```python
from build123d import *
from build123d.topology import SkipClean

# Parameters (mm, degrees)
SKETCH1_W           = 84
SKETCH1_H           = 40
BOSS_EXTRUDE1_DEPTH = 20
FILLET1_R           = 2
HOLE1_D             = 13
HOLE2_D             = 6
CUT_EXTRUDE2_DEPTH  = 17
RIB1_REACH          = 63.351
SKETCH10_WALLS_W    = 2
SKETCH10_WALLS_H    = 158.702893202
SKETCH12_W          = 3
SKETCH12_H          = 20
CUT_EXTRUDE3_DEPTH  = 60.439044407


with BuildPart() as part:
    # Sketch1 → Boss-Extrude1 (new, symmetric)
    with BuildSketch(Plane.XY):
        Rectangle(SKETCH1_W, SKETCH1_H)
    extrude(amount=BOSS_EXTRUDE1_DEPTH, both=True)

    # Fillet1
    fillet1_edges = [part.edges().sort_by_distance(p)[0] for p in [
        (42, -20, 0),
        (-42, -20, 0),
        (-42, 20, 0),
        (42, 20, 0),
    ]]
    fillet(fillet1_edges, radius=FILLET1_R)

    # Hole1 (through all)
    with Locations(Plane(origin=(0, 20, 0), x_dir=(1, 0, 0), z_dir=(0, 1, 0))):
        with Locations((0, 0)):
            Hole(HOLE1_D / 2)

    # Hole2 (through all)
    with Locations(Plane(origin=(0, 20, 0), x_dir=(1, 0, 0), z_dir=(0, 1, 0))):
        with Locations((12.5, 0), (0, -12.5), (-12.5, 0), (0, 12.5), (0, 0)):
            Hole(HOLE2_D / 2)

    # Sketch9 → Cut-Extrude2 (cut, symmetric)
    with BuildSketch(Plane(origin=(0, 0, 0), x_dir=(1, 0, 0), z_dir=(0, 1, 0))):
        with BuildLine():
            Line((-39, -20), (0, -20))
            Line((0, -20), (0, -18.5))
            ThreePointArc((0, -18.5), (-2.296100594, -18.043277195), (-4.242640687, -16.742640687))
            Line((-4.242640687, -16.742640687), (-16.742640687, -4.242640687))
            ThreePointArc((-16.742640687, -4.242640687), (-18.043277195, -2.296100594), (-18.5, 0))
            Line((-18.5, 0), (-39, 0))
            Line((-39, 0), (-39, -20))
        make_face()
        with BuildLine():
            Line((39, 0), (18.5, 0))
            ThreePointArc((18.5, 0), (18.043277195, -2.296100594), (16.742640687, -4.242640687))
            Line((16.742640687, -4.242640687), (4.242640687, -16.742640687))
            ThreePointArc((4.242640687, -16.742640687), (2.296100594, -18.043277195), (0, -18.5))
            Line((0, -18.5), (0, -20))
            Line((0, -20), (39, -20))
            Line((39, -20), (39, 0))
        make_face()
    extrude(amount=CUT_EXTRUDE2_DEPTH, both=True, mode=Mode.SUBTRACT)

    # Sketch10 walls → Rib1 (add, up to next)
    with BuildSketch(Plane.XY.offset(20), mode=Mode.PRIVATE) as rib1_sk1:
        Rectangle(SKETCH10_WALLS_W, SKETCH10_WALLS_H)
    rib1_tool1 = extrude(rib1_sk1.sketch, amount=-RIB1_REACH, mode=Mode.PRIVATE) - part.part
    # Sketch10 walls → Rib1 (add, up to next)
    with BuildSketch(Plane.XY.offset(20), mode=Mode.PRIVATE) as rib1_sk2:
        with Locations((5, 0)):
            Rectangle(SKETCH10_WALLS_W, SKETCH10_WALLS_H)
    rib1_tool2 = extrude(rib1_sk2.sketch, amount=-RIB1_REACH, mode=Mode.PRIVATE) - part.part
    # Sketch10 walls → Rib1 (add, up to next)
    with BuildSketch(Plane.XY.offset(20), mode=Mode.PRIVATE) as rib1_sk3:
        with Locations((10, 0)):
            Rectangle(SKETCH10_WALLS_W, SKETCH10_WALLS_H)
    rib1_tool3 = extrude(rib1_sk3.sketch, amount=-RIB1_REACH, mode=Mode.PRIVATE) - part.part
    # Sketch10 walls → Rib1 (add, up to next)
    with BuildSketch(Plane.XY.offset(20), mode=Mode.PRIVATE) as rib1_sk4:
        with Locations((15, 0)):
            Rectangle(SKETCH10_WALLS_W, SKETCH10_WALLS_H)
    rib1_tool4 = extrude(rib1_sk4.sketch, amount=-RIB1_REACH, mode=Mode.PRIVATE) - part.part
    # Sketch10 walls → Rib1 (add, up to next)
    with BuildSketch(Plane.XY.offset(20), mode=Mode.PRIVATE) as rib1_sk5:
        with Locations((20, 0)):
            Rectangle(SKETCH10_WALLS_W, SKETCH10_WALLS_H)
    rib1_tool5 = extrude(rib1_sk5.sketch, amount=-RIB1_REACH, mode=Mode.PRIVATE) - part.part
    # Sketch10 walls → Rib1 (add, up to next)
    with BuildSketch(Plane.XY.offset(20), mode=Mode.PRIVATE) as rib1_sk6:
        with Locations((25, 0)):
            Rectangle(SKETCH10_WALLS_W, SKETCH10_WALLS_H)
    rib1_tool6 = extrude(rib1_sk6.sketch, amount=-RIB1_REACH, mode=Mode.PRIVATE) - part.part
    # Sketch10 walls → Rib1 (add, up to next)
    with BuildSketch(Plane.XY.offset(20), mode=Mode.PRIVATE) as rib1_sk7:
        with Locations((30, 0)):
            Rectangle(SKETCH10_WALLS_W, SKETCH10_WALLS_H)
    rib1_tool7 = extrude(rib1_sk7.sketch, amount=-RIB1_REACH, mode=Mode.PRIVATE) - part.part
    # Sketch10 walls → Rib1 (add, up to next)
    with BuildSketch(Plane.XY.offset(20), mode=Mode.PRIVATE) as rib1_sk8:
        with Locations((35, 0)):
            Rectangle(SKETCH10_WALLS_W, SKETCH10_WALLS_H)
    rib1_tool8 = extrude(rib1_sk8.sketch, amount=-RIB1_REACH, mode=Mode.PRIVATE) - part.part
    # Sketch10 walls → Rib1 (add, up to next)
    with BuildSketch(Plane.XY.offset(20), mode=Mode.PRIVATE) as rib1_sk9:
        with Locations((-25, 0)):
            Rectangle(SKETCH10_WALLS_W, SKETCH10_WALLS_H)
    rib1_tool9 = extrude(rib1_sk9.sketch, amount=-RIB1_REACH, mode=Mode.PRIVATE) - part.part
    # Sketch10 walls → Rib1 (add, up to next)
    with BuildSketch(Plane.XY.offset(20), mode=Mode.PRIVATE) as rib1_sk10:
        with Locations((-20, 0)):
            Rectangle(SKETCH10_WALLS_W, SKETCH10_WALLS_H)
    rib1_tool10 = extrude(rib1_sk10.sketch, amount=-RIB1_REACH, mode=Mode.PRIVATE) - part.part
    # Sketch10 walls → Rib1 (add, up to next)
    with BuildSketch(Plane.XY.offset(20), mode=Mode.PRIVATE) as rib1_sk11:
        with Locations((-15, 0)):
            Rectangle(SKETCH10_WALLS_W, SKETCH10_WALLS_H)
    rib1_tool11 = extrude(rib1_sk11.sketch, amount=-RIB1_REACH, mode=Mode.PRIVATE) - part.part
    # Sketch10 walls → Rib1 (add, up to next)
    with BuildSketch(Plane.XY.offset(20), mode=Mode.PRIVATE) as rib1_sk12:
        with Locations((-10, 0)):
            Rectangle(SKETCH10_WALLS_W, SKETCH10_WALLS_H)
    rib1_tool12 = extrude(rib1_sk12.sketch, amount=-RIB1_REACH, mode=Mode.PRIVATE) - part.part
    # Sketch10 walls → Rib1 (add, up to next)
    with BuildSketch(Plane.XY.offset(20), mode=Mode.PRIVATE) as rib1_sk13:
        with Locations((-5, 0)):
            Rectangle(SKETCH10_WALLS_W, SKETCH10_WALLS_H)
    rib1_tool13 = extrude(rib1_sk13.sketch, amount=-RIB1_REACH, mode=Mode.PRIVATE) - part.part
    # Sketch10 walls → Rib1 (add, up to next)
    with BuildSketch(Plane.XY.offset(20), mode=Mode.PRIVATE) as rib1_sk14:
        with Locations((-30, 0)):
            Rectangle(SKETCH10_WALLS_W, SKETCH10_WALLS_H)
    rib1_tool14 = extrude(rib1_sk14.sketch, amount=-RIB1_REACH, mode=Mode.PRIVATE) - part.part
    # Sketch10 walls → Rib1 (add, up to next)
    with BuildSketch(Plane.XY.offset(20), mode=Mode.PRIVATE) as rib1_sk15:
        with Locations((-35, 0)):
            Rectangle(SKETCH10_WALLS_W, SKETCH10_WALLS_H)
    rib1_tool15 = extrude(rib1_sk15.sketch, amount=-RIB1_REACH, mode=Mode.PRIVATE) - part.part
    add(rib1_tool1.solids().sort_by_distance((0, 0, 20))[0])
    add(rib1_tool2.solids().sort_by_distance((5, 0, 20))[0])
    add(rib1_tool3.solids().sort_by_distance((10, 0, 20))[0])
    add(rib1_tool4.solids().sort_by_distance((15, 0, 20))[0])
    add(rib1_tool5.solids().sort_by_distance((20, 0, 20))[0])
    add(rib1_tool6.solids().sort_by_distance((25, 0, 20))[0])
    add(rib1_tool7.solids().sort_by_distance((30, 0, 20))[0])
    add(rib1_tool8.solids().sort_by_distance((35, 0, 20))[0])
    add(rib1_tool9.solids().sort_by_distance((-25, 0, 20))[0])
    add(rib1_tool10.solids().sort_by_distance((-20, 0, 20))[0])
    add(rib1_tool11.solids().sort_by_distance((-15, 0, 20))[0])
    add(rib1_tool12.solids().sort_by_distance((-10, 0, 20))[0])
    add(rib1_tool13.solids().sort_by_distance((-5, 0, 20))[0])
    add(rib1_tool14.solids().sort_by_distance((-30, 0, 20))[0])
    add(rib1_tool15.solids().sort_by_distance((-35, 0, 20))[0])

    # Sketch12 → Cut-Extrude3 (cut, through all)
    with SkipClean():  # the faces are left unmerged after this step: merging them gives an invalid solid
        with BuildSketch(Plane.XZ.offset(-17)):
            with Locations((37.5, 10)):
                Rectangle(SKETCH12_W, SKETCH12_H)
            with Locations((32.5, 10)):
                Rectangle(SKETCH12_W, SKETCH12_H)
            with Locations((27.5, 10)):
                Rectangle(SKETCH12_W, SKETCH12_H)
            with Locations((22.5, 10)):
                Rectangle(SKETCH12_W, SKETCH12_H)
            with BuildLine():
                Line((18.5, 0), (19, 0))
                Line((19, 0), (19, 20))
                Line((19, 20), (16, 20))
                Line((16, 20), (16, 4.985281374))
                Line((16, 4.985281374), (16.742640687, 4.242640687))
                ThreePointArc((16.742640687, 4.242640687), (18.043277195, 2.296100594), (18.5, 0))
            make_face()
            Polygon((11, 9.985281374), (14, 6.985281374), (14, 20), (11, 20), align=None)
            Polygon((6, 14.985281374), (9, 11.985281374), (9, 20), (6, 20), align=None)
            with BuildLine():
                Line((4, 16.972135955), (4, 20))
                Line((4, 20), (1, 20))
                Line((1, 20), (1, 18.416079783))
                ThreePointArc((1, 18.416079783), (2.602161303, 17.906362599), (4, 16.972135955))
            make_face()
            with BuildLine():
                Line((-4, 20), (-4, 16.972135955))
                ThreePointArc((-4, 16.972135955), (-2.602161303, 17.906362599), (-1, 18.416079783))
                Line((-1, 18.416079783), (-1, 20))
                Line((-1, 20), (-4, 20))
            make_face()
            Polygon((-9, 11.985281374), (-6, 14.985281374), (-6, 20), (-9, 20), align=None)
            Polygon((-14, 6.985281374), (-11, 9.985281374), (-11, 20), (-14, 20), align=None)
            with BuildLine():
                Line((-16.742640687, 4.242640687), (-16, 4.985281374))
                Line((-16, 4.985281374), (-16, 20))
                Line((-16, 20), (-19, 20))
                Line((-19, 20), (-19, 0))
                Line((-19, 0), (-18.5, 0))
                ThreePointArc((-18.5, 0), (-18.043277195, 2.296100594), (-16.742640687, 4.242640687))
            make_face()
            with Locations((-22.5, 10)):
                Rectangle(SKETCH12_W, SKETCH12_H)
            with Locations((-27.5, 10)):
                Rectangle(SKETCH12_W, SKETCH12_H)
            with Locations((-32.5, 10)):
                Rectangle(SKETCH12_W, SKETCH12_H)
            with Locations((-37.5, 10)):
                Rectangle(SKETCH12_W, SKETCH12_H)
        extrude(amount=-CUT_EXTRUDE3_DEPTH, mode=Mode.SUBTRACT)


solid = part.part
```
Here's how the part is built. I have some questions about the finished solid (model axes, mm). A direction names the side the tool comes from. Coordinates: 2 decimals unless noted, no trailing zeros. Write each loop counter-clockwise with the first axis right and the second up, starting at its lowest first coordinate (ties: lowest second). Pieces come first, ordered by that corner, then holes. Notation, with made-up numbers: (12, 33) -> (68, 33) arc R21 ccw to (68, 57) -> close; hole circle Ø8 at (-18, 68). An arc over 180 degrees is marked (long way). Use a Markdown table: item, result. Add a question column.
(1) If we section it at D-D, the plane y = -4: State how many separate pieces and enclosed holes the cut face has, and give its area (3 significant figures).
(2) I'm going to push flat-ended pins straight in: P1, Ø0.9, axis at x = 32.5, y = 10.5, coming from the +Z side; P2, Ø0.9, axis at x = 3, z = 18.5, coming from the +Y side. Where does each tip first touch, or does it pass through?
(3) For faces 1 (the cylindrical face through (14.9, -0.3, 1.8)), 2 (the flat face through (-28, 1, 0)), which set-ups out of +Z, -Z, +X, -X, +Y, -Y let a thin tool reach every point of the face, with its end or its side?
(4) If we section it at C-C, the plane x = -12.5: Write out the boundary of the cut face in (y, z), and give its area (3 significant figures).
(5) We'd pull the mould along X, two halves only. Please class faces 3 (the flat face through (1, 1, 19)), 4 (the flat face through (-1, 20, -9)), 5 (the flat face through (42, 0, 0)): +X half, -X half, draft (parallel to the pull), parting line (faces both ways), or undercut.
(6) If we section it at A-A, the plane z = -12.5: Write out the boundary of the cut face in (x, y), and give its area (3 significant figures).
(7) If we section it at B-B, the plane x = 0: Write out the boundary of the cut face in (y, z), and give its area (3 significant figures).
(8) Please list where these lines run through material, in increasing order: line 1 (Z direction, x = 0, y = 10); line 2 (Z direction, x = -37.5, y = -0.5); line 3 (Z direction, x = 12.5, y = -6.5).
Outcome:
| question | item | result |
|---|---|---|
| 1 | separate pieces | 1 |
| 1 | enclosed holes | 5 |
| 1 | area | 2,410 mm^2 |
| 2 | P1 | stops at z = 0 |
| 2 | P2 | stops at y = -17 |
| 3 | face 1 | +Y, -Y |
| 3 | face 2 | +Z, +Y |
| 4 | outline | (-20, -20) -> (20, -20) -> (20, -3) -> (-20, -3) -> close; (-20, 3) -> (20, 3) -> (20, 8.49) -> (-17, 8.49) -> (-17, 20) -> (-20, 20) -> close |
| 4 | area | 934 mm^2 |
| 5 | face 3 | undercut |
| 5 | face 4 | draft |
| 5 | face 5 | +X half |
| 6 | outline | (-42, -18) arc R2 ccw to (-40, -20) -> (-3, -20) -> (-3, 20) -> (-40, 20) arc R2 ccw to (-42, 18) -> close; (3, -20) -> (40, -20) arc R2 ccw to (42, -18) -> (42, 18) arc R2 ccw to (40, 20) -> (3, 20) -> close |
| 6 | area | 3,120 mm^2 |
| 7 | outline | (-20, -20) -> (20, -20) -> (20, -15.5) -> (-20, -15.5) -> close; (-20, -9.5) -> (20, -9.5) -> (20, -6.5) -> (-20, -6.5) -> close; (-20, 6.5) -> (20, 6.5) -> (20, 9.5) -> (-20, 9.5) -> close; (-20, 15.5) -> (20, 15.5) -> (20, 20) -> (-20, 20) -> close |
| 7 | area | 600 mm^2 |
| 8 | line 1 | z = -20 to -15.5, -9.5 to -6.5, 6.5 to 9.5, 15.5 to 20 |
| 8 | line 2 | z = -20 to 0 |
| 8 | line 3 | z = -20 to -3, 3 to 8.49 |
